Autodesk Fusion 360 part; units mm, degrees
sketch "Sketch1" plane through (0, 0, 0) normal (0, 0, 1) x (1, 0, 0)
  line L0 (0, 0) -> (40, 0)
  line L1 (40, 0) -> (40, 140)
  line L2 (40, 140) -> (0, 140)
  line L3 (0, 140) -> (0, 0)
  circle A0 centre (20, 130) radius 2.75
  circle A1 centre (20, 110) radius 2.75
  dimension "d1" = 40
  dimension "d2" = 140
  dimension "d3" = 5.5
  dimension "d4" = 20
  dimension "d5" = 10
  dimension "d6" = 5.5
  dimension "d7" = 20
  dimension "d8" = 20
extrude "Extrude1" add sketch "Sketch1" along normal blind 50
hole "Hole1" at (20, 130, 50) direction (0, 0, -1) diameter 10 depth 35 tip angle 180
hole "Hole2" at (20, 110, 50) direction (0, 0, -1) diameter 10 depth 35 tip angle 180
sketch "Sketch2" plane through (40, 0, 0) normal (1, 0, 0) x (0, 0, -1)
  line L0 (0, 0) -> (0, 140)
  line L1 (0, 140) -> (-50, 140)
  line L2 (-50, 140) -> (-50, 0)
  line L3 (-50, 0) -> (0, 0)
  line L4 (-50, 140) -> (-20, 140)
  line L5 (-50, 140) -> (-50, 40)
  line L6 (-50, 40) -> (-20, 140)
extrude "Extrude2" cut sketch "Sketch2" against normal blind 40 contours L1 L2 L4 L5 L6
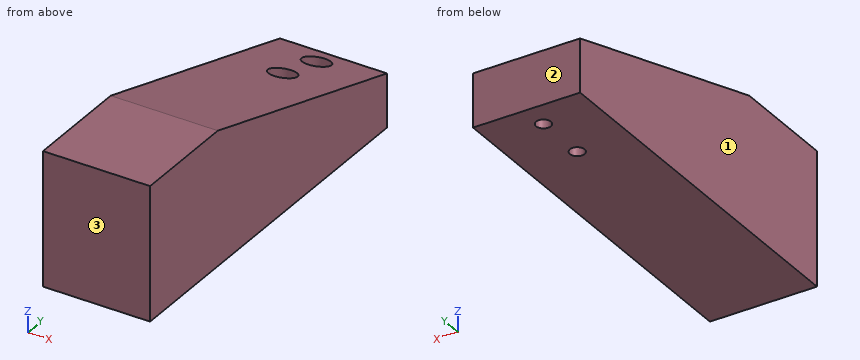
CAD build for the part. Positions are in the model's coordinates, mm. Face numbers are marked on the shaded views. Round coordinates to 2 decimals unless told otherwise and drop trailing zeros. Write each loop counter-clockwise with the first axis right and the second up, starting at its lowest first coordinate (ties: lowest second). Pieces come first, ordered by that corner, then holes. Notation, with made-up numbers: (12, -40) - (34, -40) arc R14 cw to (34, -19) - close; hole circle Ø10 at (65.5, 74.25). An arc over 180 degrees is marked (long way). Return JSON: item names as keys, results as strings. Group by question number.
Item 1: Mould opens along Y. For the marked faces 1, 2 and 3 say: +Y half, -Y half, draft (parallel to the pull), parting line (faces both ways), or undercut.
Item 2: Band-saw the part on A-A on y = 110. List the corners of the cut face in (x, z), plus the area to 4 significant figures.
Item 3: Band-saw the part on B-B on x = 20. List the corners of the cut face in (y, z).
Item 4: Band-saw the part on D-D on x = 5.5. List the corners of the cut face in (y, z).
Item 5: Flat gauge pins, fed straight in: pin 1 Ø3.5 at (x, y) = (20, 110) entering from -Z; pin 2 Ø1 at (x, y) = (25, 88.5) entering from +Z; pin 3 Ø8 at (x, y) = (18, 111.5) entering from +Z; pin 4 Ø3 at (x, z) = (22.5, 23.5) entering from +Y. Where does each tip first touch, or does it go through?
Item 6: Band-saw the part on C-C on y = 130. List the corners of the cut face in (x, z), plus the area to 4 significant figures.
Item 7: Probe probe 1 along Y at (x, z) = (20, 3.5); probe 2 along Y at (x, z) = (20, 18); probe 3 along X at (y, z) = (130, 4). List the from-to ranges inside material, lowest first.
Resolved:
{
 "1": {"face 1": "draft", "face 2": "+Y half", "face 3": "-Y half"},
 "2": {"outline": "(0, 0) - (17.25, 0) - (17.25, 15) - (15, 15) - (15, 29) - (0, 29) - close; (22.75, 0) - (40, 0) - (40, 29) - (25, 29) - (25, 15) - (22.75, 15) - close", "area": "937.5 mm²"},
 "3": {"outline": "(0, 0) - (107.25, 0) - (107.25, 15) - (105, 15) - (105, 30.5) - (40, 50) - (0, 50) - close; (112.75, 0) - (127.25, 0) - (127.25, 15) - (125, 15) - (125, 24.5) - (115, 27.5) - (115, 15) - (112.75, 15) - close; (132.75, 0) - (140, 0) - (140, 20) - (135, 21.5) - (135, 15) - (132.75, 15) - close"},
 "4": {"outline": "(0, 0) - (140, 0) - (140, 20) - (40, 50) - (0, 50) - close"},
 "5": {"pin 1": "passes through", "pin 2": "stops at z = 35.6", "pin 3": "stops at z = 29.4", "pin 4": "stops at y = 127"},
 "6": {"outline": "(0, 0) - (17.25, 0) - (17.25, 15) - (15, 15) - (15, 23) - (0, 23) - close; (22.75, 0) - (40, 0) - (40, 23) - (25, 23) - (25, 15) - (22.75, 15) - close", "area": "757.5 mm²"},
 "7": {"probe 1": "y = 0 to 107.25, 112.75 to 127.25, 132.75 to 140", "probe 2": "y = 0 to 105, 115 to 125, 135 to 140", "probe 3": "x = 0 to 17.25, 22.75 to 40"}
}
